```python
from build123d import *

# Parameters (mm, degrees)
SKETCH1_R           = 5.98
BOSS_EXTRUDE1_DEPTH = 5
SKETCH2_R           = 1.25
CUT_EXTRUDE1_DEPTH  = 5
SKETCH3_R           = 5.75
BOSS_EXTRUDE2_DEPTH = 3
SKETCH4_R           = 5.98
BOSS_EXTRUDE3_DEPTH = 2.62
SKETCH5_R           = 0.645
BOSS_EXTRUDE4_DEPTH = 7
SKETCH6_R           = 0.645
SKETCH6_R_2         = 0.3
CUT_EXTRUDE2_DEPTH  = 7


with BuildPart() as part:
    # Sketch1 → Boss-Extrude1 (new body)
    with BuildSketch(Plane.XY):
        Circle(SKETCH1_R)
    extrude(amount=BOSS_EXTRUDE1_DEPTH)

    # Sketch2 → Cut-Extrude1 (cut)
    with BuildSketch(Plane(origin=(0, 0, 0), x_dir=(-1, 0, 0), z_dir=(0, 0, -1))):
        Circle(SKETCH2_R)
    extrude(amount=-CUT_EXTRUDE1_DEPTH, mode=Mode.SUBTRACT)

    # Sketch3 → Boss-Extrude2 (add)
    with BuildSketch(Plane.XY.offset(5)):
        Circle(SKETCH3_R)
    extrude(amount=BOSS_EXTRUDE2_DEPTH)

    # Sketch4 → Boss-Extrude3 (add)
    with BuildSketch(Plane.XY.offset(8)):
        Circle(SKETCH4_R)
    extrude(amount=BOSS_EXTRUDE3_DEPTH)

    # Sketch5 → Boss-Extrude4 (add)
    with BuildSketch(Plane.XY.offset(10.62)):
        with Locations((-2.5, 0)):
            Circle(SKETCH5_R)
        with Locations((2.5, 0)):
            Circle(SKETCH5_R)
    extrude(amount=BOSS_EXTRUDE4_DEPTH)

    # Sketch6 → Cut-Extrude2 (cut)
    with BuildSketch(Plane.XY.offset(17.62)):
        with Locations((-2.5, 0)):
            Circle(SKETCH6_R)
        with Locations((-2.5, 0)):
            Circle(SKETCH6_R_2, mode=Mode.SUBTRACT)
        with Locations((2.5, 0)):
            Circle(SKETCH6_R)
        with Locations((2.5, 0)):
            Circle(SKETCH6_R_2, mode=Mode.SUBTRACT)
    extrude(amount=-CUT_EXTRUDE2_DEPTH, mode=Mode.SUBTRACT)


solid = part.part
```
Read the model definition and answer for the solid it produces. Units are mm, in the model's axes. A direction names the side the tool comes from. Give positions to 0.01 mm unless a question says otherwise; leave off trailing zeros. Write each loop counter-clockwise with the first axis right and the second up, starting at its lowest first coordinate (ties: lowest second). Pieces come first, ordered by that corner, then holes. Notation, with made-up numbers: M 32.5,18.5 L 38.5,18.5 A31 ccw 38.5,45.5 Z; hole C 56,48.25 d7. An arc over 180 degrees is marked long. Put each result on its own line as item: value. Start each with the question number.
1. The part is cut by section C-C, the plane z = 11.5. Give the vertices of the cut face in (x, y), and give its area (3 significant figures).
2. Which of the six approach directions +Z, -Z, +X, -X, +Y, -Y give full straight-line access (tool end or side, diameter ignored) to faces 5 (the flat face through (0, 0, 5)), 6 (the cylindrical face through (2.759, -5.305, 2.465))?
3. The part is cut by section D-D, the plane z = 2.25. Give the vertices of the cut face in (x, y), and give its area (3 significant figures).
4. The part is cut by section A-A, the plane y = 0. Give the vertices of the cut face in (x, z), and give its area (3 significant figures).
5. Consider line 1 along Y through (x, z) = (0, 2.6); line 2 along Z through (x, y) = (5, -0.75); line 3 along X through (y, z) = (0.5, 1.5). Determine where each line is inside the solid, lowest interval first.
6. Each of these flat-tipped pins is pushed along its axis until it touches: pin 1 Ø1 at (x, y) = (0.5, 1) entering from +Z; pin 2 Ø1.2 at (x, y) = (0, 0.5) entering from -Z; pin 3 Ø3 at (y, z) = (2, 7) entering from -X. Where does it stop, or does it pass through?
7. For a pull along Z with two mould halves and no side action, classify faces 1 (the flat face through (-0.1, 1.4, 0)), 2 (the cylindrical face through (-0.75, 5.7, 6.48)), 3 (the flat face through (0, 0, 10.62)), 4 (the cylindrical face through (0.27, -1.22, 2.46)) as released by +Z, released by -Z, zero draft, split by the parting line, or undercut.
8. The part is cut by section B-B, the plane x = 0. Give the vertices of the cut face in (y, z).
Final values:
1. outline: C -2.5,0 d0.6; C 2.5,0 d0.6
1. area: 0.565 mm²
2. face 5: -Z
2. face 6: +Z, -Z
3. outline: C 0,0 d11.96; hole C 0,0 d2.5
3. area: 107 mm²
4. outline: M -5.98,0 L -1.25,0 L -1.25,5 L 1.25,5 L 1.25,0 L 5.98,0 L 5.98,5 L 5.75,5 L 5.75,8 L 5.98,8 L 5.98,10.62 L 2.8,10.62 L 2.8,17.62 L 2.2,17.62 L 2.2,10.62 L -2.2,10.62 L -2.2,17.62 L -2.8,17.62 L -2.8,10.62 L -5.98,10.62 L -5.98,8 L -5.75,8 L -5.75,5 L -5.98,5 Z
4. area: 122 mm²
5. line 1: y = -5.98 to -1.25, 1.25 to 5.98
5. line 2: z = 0 to 10.62
5. line 3: x = -5.96 to -1.15, 1.15 to 5.96
6. pin 1: stops at z = 10.62
6. pin 2: stops at z = 5
6. pin 3: stops at x = -5.91
7. face 1: released by -Z
7. face 2: undercut
7. face 3: released by +Z
7. face 4: zero draft
8. outline: M -5.98,0 L -1.25,0 L -1.25,5 L 1.25,5 L 1.25,0 L 5.98,0 L 5.98,5 L 5.75,5 L 5.75,8 L 5.98,8 L 5.98,10.62 L -5.98,10.62 L -5.98,8 L -5.75,8 L -5.75,5 L -5.98,5 Z
